The drawing under review shows one solid part. Ordinate dimensions are in mm from its lowest x, y, z. A direction names the side the tool comes from. Coordinates: 2 decimals unless noted, no trailing zeros. Order: outer loops, then holes, each group sorted by start corner. A loop starts at its lowest first (then second) coordinate and runs counter-clockwise, first axis right, second up.
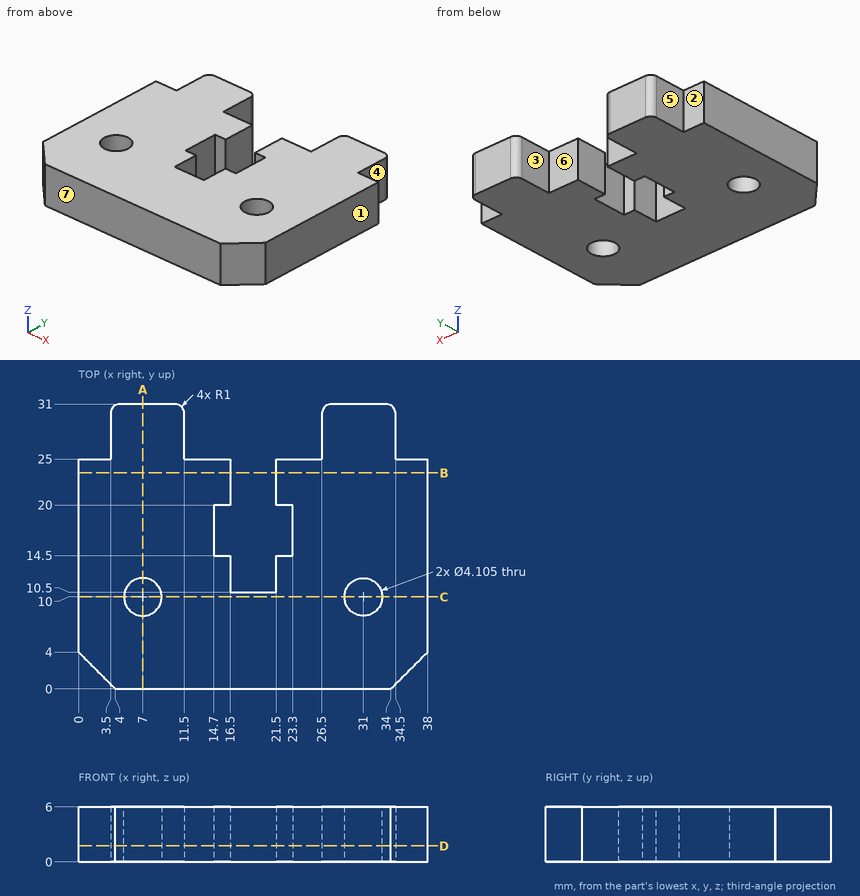
(1) Consider section C-C (y = 10). Give the boundary of the cut face in (x, z), then the cut area to 3 significant figures.
(2) Tool access review of the marked faces 4, 5, 6 and 7: name each direction out of +Z, -Z, +X, -X, +Y, -Y from which nothing blocks a thin tool from reaching the whole face with its end or side.
(3) Consider section B-B (y = 23.5). Give the boundary of the cut face in (x, z), then the cut area to 3 significant figures.
(4) Insertion check: pin 1 Ø1.5 at (x, z) = (23.5, 3.5) entering from +Y; pin 2 Ø2.5 at (x, z) = (20, 2.5) entering from +Y; pin 3 Ø2.5 at (y, z) = (27, 2) entering from +X. Each pin has a flat end and moves straight along its axis. Give the tip position at first contact, or say it passes through.
(5) Wall thickness on line 1 (X direction, y = 15, z = 0.75); line 2 (Y direction, x = 31, z = 3.35); line 3 (X direction, y = 9, z = 1.75): over which ranges is each line inside the solid? List them lowest first.
(6) Consider section D-D (z = 1.75). Give the number of separate pieces and of enclosed holes in the cut face, then the cut area to 3 significant figures.
(7) The part is to be moulded in two halves that separate along X. For the marked faces 1, 2 and 3, say which applies: +X half, -X half, draft (parallel to the pull), parting line (faces both ways), or undercut.
(8) Consider section A-A (x = 7). Give the boundary of the cut face in (y, z), then the cut area to 3 significant figures.
Findings:
1. outline: (0, 0) - (4.95, 0) - (4.95, 6) - (0, 6) - close; (9.05, 0) - (28.95, 0) - (28.95, 6) - (9.05, 6) - close; (33.05, 0) - (38, 0) - (38, 6) - (33.05, 6) - close
1. area: 179 mm2
2. face 4: +Z, -Z, +X, +Y
2. face 5: +Z, -Z, -X, +Y
2. face 6: +Z, -Z, +Y
2. face 7: +Z, -Z, +X, -X, -Y
3. outline: (0, 0) - (16.5, 0) - (16.5, 6) - (0, 6) - close; (21.5, 0) - (38, 0) - (38, 6) - (21.5, 6) - close
3. area: 198 mm2
4. pin 1: stops at y = 25
4. pin 2: stops at y = 10.5
4. pin 3: stops at x = 34.5
5. line 1: x = 0 to 14.7, 23.3 to 38
5. line 2: y = 0 to 7.95, 12.05 to 31
5. line 3: x = 0 to 5.21, 8.79 to 29.21, 32.79 to 38
6. separate pieces: 1
6. enclosed holes: 2
6. area: 910 mm2
7. face 1: +X half
7. face 2: draft
7. face 3: undercut
8. outline: (0, 0) - (7.95, 0) - (7.95, 6) - (0, 6) - close; (12.05, 0) - (31, 0) - (31, 6) - (12.05, 6) - close
8. area: 161 mm2
